The model under review builds one solid part; all positions refer to its coordinate system, in mm. Round coordinates to 2 decimals unless told otherwise and drop trailing zeros. Write each loop counter-clockwise with the first axis right and the second up, starting at its lowest first coordinate (ties: lowest second). Pieces come first, ordered by that corner, then holes. Notation, with made-up numbers: (14, 80.25) -> (42, 80.25) arc R29 cw to (42, 115.25) -> close; hole circle Ø5 at (-5, 23.25). An arc over 180 degrees is marked (long way). Return JSON: item names as keys, results as strings. Group by question number.
1. Clearance check with flat-ended pins moving along their axes: P1, Ø0.8, axis at x = 1, z = 44, coming from the -Y side (3 decimals); P2, Ø0.8, axis at x = 1, y = -4.5, coming from the +Z side; P3, Ø1.3, axis at x = 1.5, z = -45, coming from the +Y side (3 decimals). State where each tip first meets the part, or that it passes through.
2. Take a section at D-D, the plane y = 3.75. Write out the cut boundary in (x, z), then the cut area to 3 significant figures.
3. Take a section at A-A, the plane y = -2.75. Write out the cut boundary in (x, z), then the cut area to 3 significant figures.
4. Take a section at B-B, the plane x = 1.75. Write out the cut boundary in (y, z) (3 decimals), then the cut area to 3 significant figures.
5. Take a section at C-C, the plane z = -7. Write out the cut boundary in (x, y), then the cut area to 3 significant figures.
6. For line 1 along Z through (x, y) = (0.5, -4.25); line 2 along Z through (x, y) = (1.55, -1); line 3 along Y through (x, z) = (1.15, 2), list the stretches that pass through material, from the lowest coordinate up. Write a range as from..to.
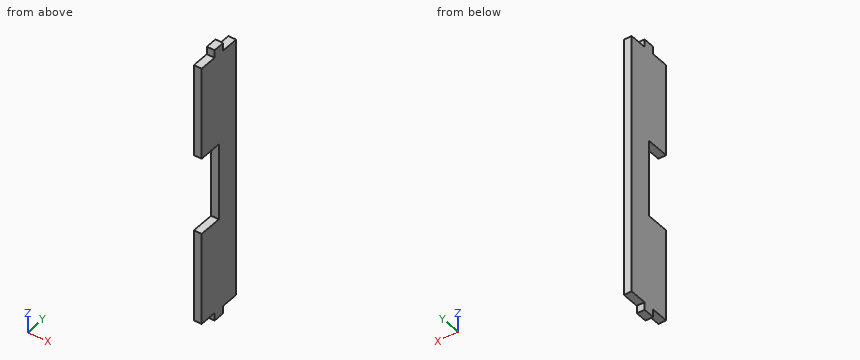
from build123d import *

# Parameters (mm, degrees)
BOSS_EXTRUDE1_DEPTH = 2.54
CUT_EXTRUDE1_REACH  = 4.54
SKETCH2_W           = 25.4
SKETCH2_H           = 7.62


with BuildPart() as part:
    # Sketch1 → Boss-Extrude1 (new body)
    with BuildSketch(Plane(origin=(0, 0, 0), x_dir=(0, 0, -1), z_dir=(1, 0, 0))):
        Polygon((-43.18, 7.62), (-43.18, 1.905), (-45.72, 1.905), (-45.72, -1.905), (-43.18, -1.905), (-43.18, -7.62), (43.18, -7.62), (43.18, -1.905), (45.72, -1.905), (45.72, 1.905), (43.18, 1.905), (43.18, 7.62), align=None)
    extrude(amount=BOSS_EXTRUDE1_DEPTH)

    # Sketch2 → Cut-Extrude1 (cut, up to next)
    with BuildSketch(Plane(origin=(2.54, 0, 0), x_dir=(0, 0, -1), z_dir=(1, 0, 0)), mode=Mode.PRIVATE) as cut_extrude1_sk1:
        with Locations((0, -3.81)):
            Rectangle(SKETCH2_W, SKETCH2_H)
    cut_extrude1_tool1 = extrude(cut_extrude1_sk1.sketch, amount=-CUT_EXTRUDE1_REACH, mode=Mode.PRIVATE) & part.part
    add(cut_extrude1_tool1.solids().sort_by_distance((2.54, -3.81, 0))[0], mode=Mode.SUBTRACT)


solid = part.part
Output:
{
 "1": {"P1": "stops at y = -1.905", "P2": "stops at z = 43.18", "P3": "stops at y = 1.905"},
 "2": {"outline": "(0, -43.18) -> (2.54, -43.18) -> (2.54, 43.18) -> (0, 43.18) -> close", "area": "219 mm^2"},
 "3": {"outline": "(0, -43.18) -> (2.54, -43.18) -> (2.54, -12.7) -> (0, -12.7) -> close; (0, 12.7) -> (2.54, 12.7) -> (2.54, 43.18) -> (0, 43.18) -> close", "area": "155 mm^2"},
 "4": {"outline": "(-7.62, -43.18) -> (-1.905, -43.18) -> (-1.905, -45.72) -> (1.905, -45.72) -> (1.905, -43.18) -> (7.62, -43.18) -> (7.62, 43.18) -> (1.905, 43.18) -> (1.905, 45.72) -> (-1.905, 45.72) -> (-1.905, 43.18) -> (-7.62, 43.18) -> (-7.62, 12.7) -> (0, 12.7) -> (0, -12.7) -> (-7.62, -12.7) -> close", "area": "1,140 mm^2"},
 "5": {"outline": "(0, 0) -> (2.54, 0) -> (2.54, 7.62) -> (0, 7.62) -> close", "area": "19.4 mm^2"},
 "6": {"line 1": "z = -43.18..-12.7, 12.7..43.18", "line 2": "z = -45.72..-12.7, 12.7..45.72", "line 3": "y = 0..7.62"}
}
